Input: dimensioned drawing with shaded views. Units: mm. Origin: part minimum x, y, z. A direction names the side the tool comes from. Round coordinates to 2 decimals unless told otherwise and drop trailing zeros. Loops run counter-clockwise (first coordinate to the right, second up) from the corner with the lowest first, then second, coordinate; pieces in that order, holes last. Notation, with made-up numbers: M -7,86.5 L 33,86.5 A26 cw 33,116.5 Z; hole C 70.5,-26.75 d4. An arc over 180 degrees is marked long. Write each question's results on one line, items separated by ' | '. Start each with the question number.
1. Section D-D on x = 65.5. Output: boundary loops of the cut face in (y, z).
2. Section A-A on y = 13.5. Output: boundary loops of the cut face in (x, z), and give its area (3 significant figures).
3. Ray query, line 1 (X direction, y = 1.3, z = 91); line 2 (X direction, y = 5, z = 90). Return the intervals inside material, ascending.
4. Section B-B on x = 18. Output: boundary loops of the cut face in (y, z).
5. Set-up query: the marked faces 4 and 5. Return all of +Z, -Z, +X, -X, +Y, -Y with unobstructed straight access to the full face (end or side cutting, diameter ignored); none if empty.
6. Section C-C on z = 91. Output: boundary loops of the cut face in (x, y), and give its area (3 significant figures).
7. Draft query along Z for the marked faces 1, 2 and 3. Return one class per face: released by +Z, released by -Z, zero draft, split by the parting line, or undercut.
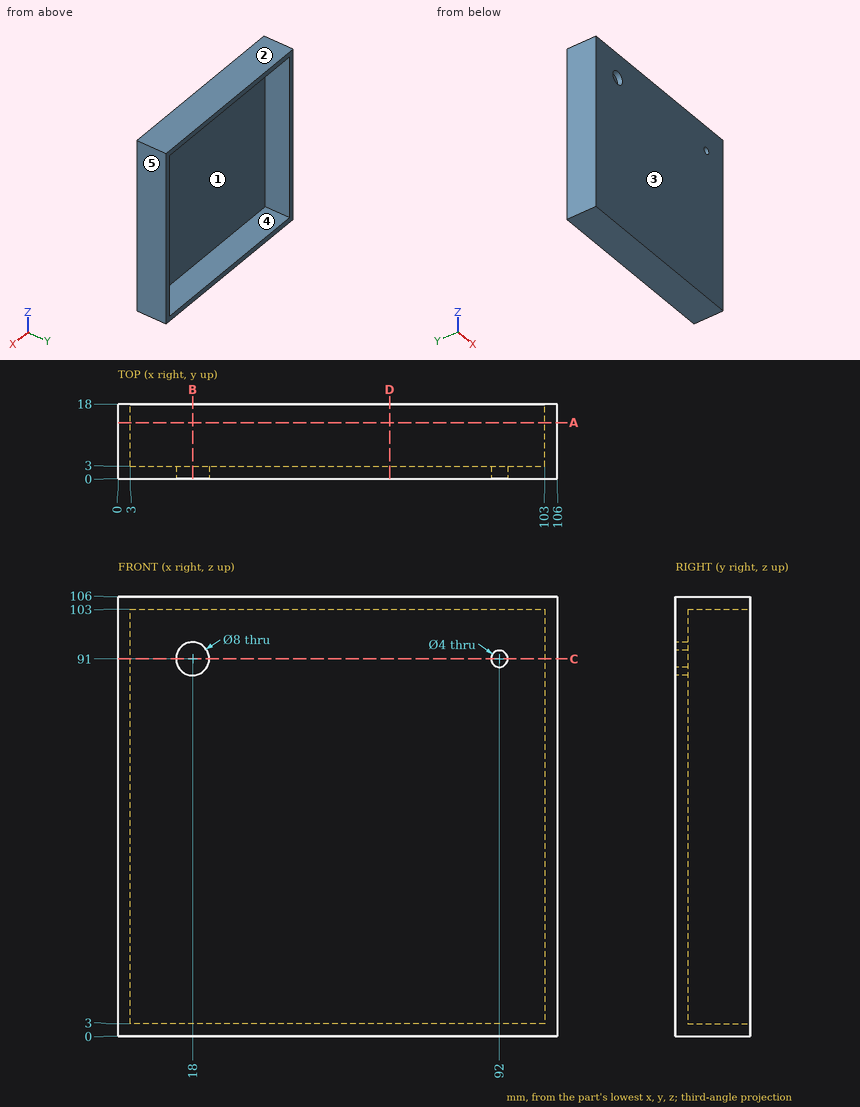
Taken from the geometry:
1) outline: M 0,0 L 18,0 L 18,3 L 3,3 L 3,103 L 18,103 L 18,106 L 0,106 Z
2) outline: M 0,0 L 106,0 L 106,106 L 0,106 Z; hole M 3,3 L 103,3 L 103,103 L 3,103 Z | area: 1,240 mm^2
3) line 1: 0 to 14, 22 to 90, 94 to 106 | line 2: 0 to 3, 103 to 106
4) outline: M 0,0 L 18,0 L 18,3 L 3,3 L 3,87 L 0,87 Z; M 0,95 L 3,95 L 3,103 L 18,103 L 18,106 L 0,106 Z
5) face 4: +Y | face 5: +Z, -Z, +X, +Y, -Y
6) outline: M 0,0 L 14,0 L 14,3 L 3,3 L 3,18 L 0,18 Z; M 22,0 L 90,0 L 90,3 L 22,3 Z; M 94,0 L 106,0 L 106,18 L 103,18 L 103,3 L 94,3 Z | area: 372 mm^2
7) face 1: undercut | face 2: released by +Z | face 3: zero draft
